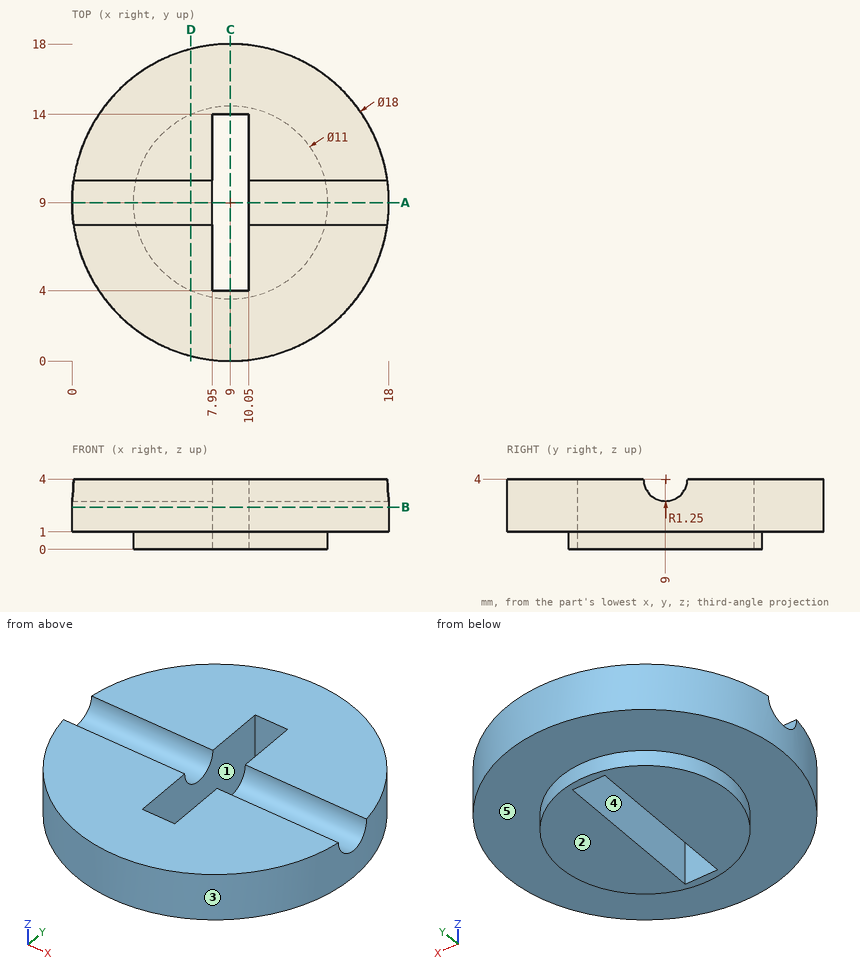
Part print with two shaded views. Sizes in mm from the minimum x, y, z corner. A direction names the side the tool comes from. Round coordinates to 2 decimals unless told otherwise and drop trailing zeros. Loops run counter-clockwise (first coordinate to the right, second up) from the corner with the lowest first, then second, coordinate; pieces in that order, holes last. Notation, with made-up numbers: M 14.25,41 L 48.25,41 A21 ccw 48.25,68 Z; hole C -26.75,56.25 d1. An arc over 180 degrees is marked long. Return JSON: item names as keys, results as strings. Group by question number.
(1) Wall check: probe 1 along Y at (x, z) = (10.75, 3.85); probe 2 along X at (y, z) = (7.5, 1.95); probe 3 along X at (y, z) = (13.5, 0.4). Give the ranges that are in metal, low to high. Write a range as [from, to].
(2) Drop flat-ended pins along their axis: P1, Ø2, axis at y = 11.5, z = 1, coming from the -X side; P2, Ø2, axis at y = 13, z = 1.5, coming from the +X side. Give the stop position or say it passes through.
(3) Saw through at B-B, the plane z = 2.4. List the corners of the cut face in (x, y), and give its area (3 significant figures).
(4) Saw through at A-A, the plane y = 9. List the corners of the cut face in (x, z).
(5) Mould opens along X. For the marked faces 3, 4 and 5 say: +X half, -X half, draft (parallel to the pull), parting line (faces both ways), or undercut.
(6) Saw through at C-C, the plane x = 9. List the corners of the cut face in (y, z).
(7) Saw through at D-D, the plane x = 6.75. List the corners of the cut face in (y, z), and give its area (3 significant figures).
(8) Tool access for the marked faces 1 and 2: list every direction of +Z, -Z, +X, -X, +Y, -Y with a clear straight run to the whole face (end or side of a thin tool).
Answer list:
{
 "1": {"probe 1": "[0.17, 7.76], [10.24, 17.83]", "probe 2": "[0.13, 7.95], [10.05, 17.87]", "probe 3": "[5.84, 7.95], [10.05, 12.16]"},
 "2": {"P1": "x = 0.13", "P2": "x = 17.49"},
 "3": {"outline": "C 9,9 d18; hole M 7.95,4 L 10.05,4 L 10.05,14 L 7.95,14 Z", "area": "233 mm2"},
 "4": {"outline": "M 0,1 L 3.5,1 L 3.5,0 L 7.95,0 L 7.95,2.75 L 0,2.75 Z; M 10.05,0 L 14.5,0 L 14.5,1 L 18,1 L 18,2.75 L 10.05,2.75 Z"},
 "5": {"face 3": "parting line", "face 4": "undercut", "face 5": "draft"},
 "6": {"outline": "M 0,1 L 3.5,1 L 3.5,0 L 4,0 L 4,4 L 0,4 Z; M 14,0 L 14.5,0 L 14.5,1 L 18,1 L 18,4 L 14,4 Z"},
 "7": {"outline": "M 0.29,1 L 3.98,1 L 3.98,0 L 14.02,0 L 14.02,1 L 17.71,1 L 17.71,4 L 10.25,4 A1.25 cw 7.75,4 L 0.29,4 Z", "area": "59.9 mm2"},
 "8": {"face 1": "+Z, -Z", "face 2": "-Z, +X, -X, +Y, -Y"}
}
